Source: CAD feature listing. Evaluate the final solid. Frame: model axes, mm. Face numbers are marked on the shaded views. Round coordinates to 2 decimals unless told otherwise and drop trailing zeros. Write each loop counter-clockwise with the first axis right and the second up, starting at its lowest first coordinate (ties: lowest second). Pieces come first, ordered by that corner, then holes. Notation, with made-up numbers: M 31,6.25 L 67,6.25 A30 ccw 67,44.25 Z; hole C 18.25,14 d8. An arc over 180 degrees is marked long. Answer in a Markdown table with one row per item.
Autodesk Inventor part; units mm, degrees
ref_plane "YZ Plane" through (0, 0, 0) normal (1, 0, 0) x (0, 1, 0)
ref_plane "XZ Plane" through (0, 0, 0) normal (0, 1, 0) x (-1, 0, 0)
ref_plane "XY Plane" through (0, 0, 0) normal (0, 0, 1) x (1, 0, 0)
sketch "Sketch1" plane through (0, 0, 0) normal (0, 0, 1) x (1, 0, 0)
  line L0 (0, -5.0856) -> (0, -49.3)
  line L1 (0, -54.8) -> (-50, -54.8)
  line L2 (-50, -5.0856) -> (-50, -49.3)
  line L3 (-5.3931, 0) -> (-44.6069, 0)
  line L4 (-50, -27.1928) -> (0, -27.1928) construction
  line L5 (-25, 0) -> (-25, -54.8) construction
  line L6 (-55, 5.1) -> (5, 5.1)
  line L7 (5, 5.1) -> (5, -59.9)
  line L8 (5, -59.9) -> (-55, -59.9)
  line L9 (-55, -59.9) -> (-55, 5.1)
  line L10 (-55, 5.1) -> (5, -59.9) construction
  line L11 (5, 5.1) -> (-55, -59.9) construction
  point P0 (0, 0)
  point P1 (-25, -27.4)
  dimension "d0" = 60
  dimension "d1" = 65
extrude "Extrusion1" add sketch "Sketch1" along normal blind 6
sketch "Sketch2" plane through (0, 0, 6) normal (0, 0, 1) x (1, 0, 0)
  circle A0 centre (-40, -11) radius 2
  circle A1 centre (-40, -26) radius 2
  circle A2 centre (-40, -41) radius 2
  circle A3 centre (-10, -41) radius 2
  circle A4 centre (-10, -26) radius 2
  circle A5 centre (-10, -11) radius 2
  point P0 (0, 0)
extrude "Extrusion2" cut sketch "Sketch2" against normal blind 6
fillet "Fillet1" radius 5 4 edges at (-55, -59.9, 3) (-55, 5.1, 3) (5, -59.9, 3) (5, 5.1, 3)
properties part number "Wheel height spacers"
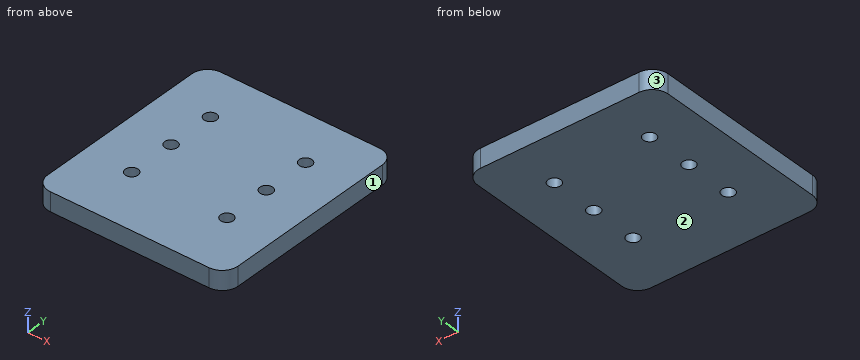
Q1. Material intervals for probe 1 along Y at (x, z) = (-40, 1.6); probe 2 along X at (y, z) = (-56, 3.15), sorted ascending.
Solutions:
| item | result |
|---|---|
| probe 1 | y = -59.9 to -43, -39 to -28, -24 to -13, -9 to 5.1 |
| probe 2 | x = -54.88 to 4.88 |
Q2. Pull-direction query (X, two-part tool) for the marked faces 1, 2 and 3; classes: pulls with the +X half, pulls with the -X half, needs draft (parallel to the pull), parting line crosses it, or undercut.
Solutions:
| item | result |
|---|---|
| face 1 | pulls with the +X half |
| face 2 | needs draft |
| face 3 | pulls with the -X half |
Q3. Section B-B (y = -11). Return loops of the section in (x, z), and give its area (3 significant figures).
Solutions:
| item | result |
|---|---|
| outline | M -55,0 L -42,0 L -42,6 L -55,6 Z; M -38,0 L -12,0 L -12,6 L -38,6 Z; M -8,0 L 5,0 L 5,6 L -8,6 Z |
| area | 312 mm2 |
Q4. Section A-A (x = -10). Return loops of the section in (y, z).
Solutions:
| item | result |
|---|---|
| outline | M -59.9,0 L -43,0 L -43,6 L -59.9,6 Z; M -39,0 L -28,0 L -28,6 L -39,6 Z; M -24,0 L -13,0 L -13,6 L -24,6 Z; M -9,0 L 5.1,0 L 5.1,6 L -9,6 Z |
Q5. Contact query for a flat-ended pin moving along its axis: pin 1 Ø3 at (x, y) = (-40, -26) entering from +Z. Output: stop coordinate, or through.
Solutions:
| item | result |
|---|---|
| pin 1 | passes through |
Q6. Section C-C (z = 4.95). Return loops of the section in (x, y), and give its area (3 significant figures).
Solutions:
| item | result |
|---|---|
| outline | M -55,-54.9 A5 ccw -50,-59.9 L 0,-59.9 A5 ccw 5,-54.9 L 5,0.1 A5 ccw 0,5.1 L -50,5.1 A5 ccw -55,0.1 Z; hole C -40,-41 d4; hole C -40,-26 d4; hole C -40,-11 d4; hole C -10,-41 d4; hole C -10,-26 d4; hole C -10,-11 d4 |
| area | 3,800 mm2 |
